from build123d import *

# Parameters (mm, degrees)
SKETCH1_W             = 203.2
SKETCH1_H             = 127
BOSS_EXTRUDE1_DEPTH   = 6.35
SKETCH2_W             = 196.85
SKETCH2_H             = 120.65
CUT_EXTRUDE1_DEPTH    = 7.35
SKETCH4_W             = 234.95
SKETCH4_H             = 158.75
SKETCH4_W_2           = 203.2
SKETCH4_H_2           = 127
BOSS_EXTRUDE2_DEPTH   = 6.35
SKETCH7_W             = 215.6206
SKETCH7_H             = 139.4206
SKETCH7_W_2           = 206.375
SKETCH7_H_2           = 130.175
CUT_EXTRUDE2_DEPTH    = 2.6416
F_8_32_TAPPED_HOLE1_D = 3.4544
FILLET3_R             = 4.6228
FILLET4_R             = 9.2456
FILLET5_R             = 3.175
F_6_CLEARANCE_HOLE1_D = 3.7973
SKETCH18_W            = 203.2
SKETCH18_H            = 127
CUT_EXTRUDE3_DEPTH    = 3.175
FILLET6_R             = 3.175


with BuildPart() as part:
    # Sketch1 → Boss-Extrude1 (new body)
    with BuildSketch(Plane(origin=(0, 0, 0), x_dir=(1, 0, 0), z_dir=(0, 1, 0))):
        Rectangle(SKETCH1_W, SKETCH1_H)
    extrude(amount=BOSS_EXTRUDE1_DEPTH)

    # Sketch2 → Cut-Extrude1 (cut, through all)
    with BuildSketch(Plane(origin=(0, 6.35, 0), x_dir=(1, 0, 0), z_dir=(0, 1, 0))):
        Rectangle(SKETCH2_W, SKETCH2_H)
    extrude(amount=-CUT_EXTRUDE1_DEPTH, mode=Mode.SUBTRACT)

    # Sketch4 → Boss-Extrude2 (add)
    with BuildSketch(Plane(origin=(0, 6.35, 0), x_dir=(1, 0, 0), z_dir=(0, 1, 0))):
        Rectangle(SKETCH4_W, SKETCH4_H)
        Rectangle(SKETCH4_W_2, SKETCH4_H_2, mode=Mode.SUBTRACT)
    extrude(amount=-BOSS_EXTRUDE2_DEPTH)

    # Sketch7 → Cut-Extrude2 (cut)
    with BuildSketch(Plane(origin=(0, 6.35, 0), x_dir=(1, 0, 0), z_dir=(0, 1, 0))):
        Rectangle(SKETCH7_W, SKETCH7_H)
        Rectangle(SKETCH7_W_2, SKETCH7_H_2, mode=Mode.SUBTRACT)
    extrude(amount=-CUT_EXTRUDE2_DEPTH, mode=Mode.SUBTRACT)

    # #8-32 Tapped Hole1 (through all)
    with Locations(Plane(origin=(0, 6.35, 0), x_dir=(1, 0, 0), z_dir=(0, 1, 0))):
        with Locations((56.321325, 74.54265), (112.64265, 74.54265), (112.64265, 24.84755), (0, 74.54265), (112.64265, -24.84755), (112.64265, -74.54265), (56.321325, -74.54265), (0, -74.54265), (-56.321325, -74.54265), (-112.64265, -74.54265), (-112.64265, -24.84755), (-112.64265, 24.84755), (-112.64265, 74.54265), (-56.321325, 74.54265)):
            Hole(F_8_32_TAPPED_HOLE1_D / 2)

    # Fillet3
    fillet3_edges = [part.edges().sort_by_distance(p)[0] for p in [
        (-103.1875, 5.0292, -65.0875),
        (103.1875, 5.0292, -65.0875),
        (103.1875, 5.0292, 65.0875),
        (-103.1875, 5.0292, 65.0875),
    ]]
    fillet(fillet3_edges, radius=FILLET3_R)

    # Fillet4
    fillet4_edges = [part.edges().sort_by_distance(p)[0] for p in [
        (-107.8103, 5.0292, -69.7103),
        (107.8103, 5.0292, -69.7103),
        (107.8103, 5.0292, 69.7103),
        (-107.8103, 5.0292, 69.7103),
    ]]
    fillet(fillet4_edges, radius=FILLET4_R)

    # Fillet5
    fillet5_edges = [part.edges().sort_by_distance(p)[0] for p in [
        (-98.425, 3.175, -60.325),
        (98.425, 3.175, -60.325),
        (98.425, 3.175, 60.325),
        (-98.425, 3.175, 60.325),
    ]]
    fillet(fillet5_edges, radius=FILLET5_R)

    # #6 Clearance Hole1 (through all)
    with Locations(Plane(origin=(0, 0, 0), x_dir=(-1, 0, 0), z_dir=(0, -1, 0))):
        with Locations((-98.425, 74.54265), (-98.425, -74.54265), (98.425, -74.54265), (98.425, 74.54265)):
            Hole(F_6_CLEARANCE_HOLE1_D / 2)

    # Sketch18 → Cut-Extrude3 (cut)
    with BuildSketch(Plane.XZ):
        Rectangle(SKETCH18_W, SKETCH18_H)
    extrude(amount=-CUT_EXTRUDE3_DEPTH, mode=Mode.SUBTRACT)

    # Fillet6
    fillet6_edges = [part.edges().sort_by_distance(p)[0] for p in [
        (-101.6, 1.5875, -63.5),
        (-101.6, 1.5875, 63.5),
        (101.6, 1.5875, 63.5),
        (101.6, 1.5875, -63.5),
    ]]
    fillet(fillet6_edges, radius=FILLET6_R)


solid = part.part
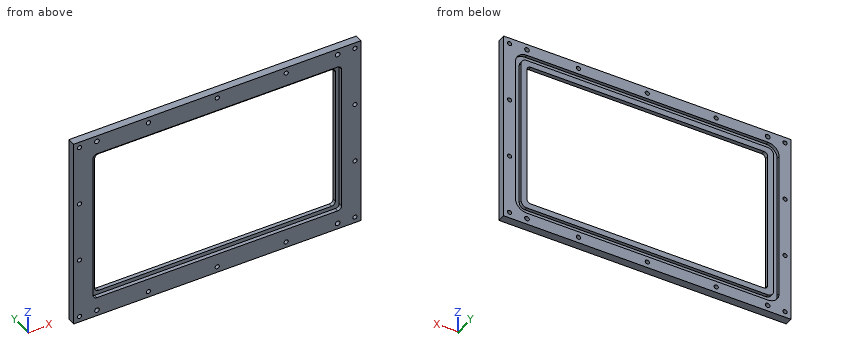
Here's how the part is built. I have some questions about the finished solid (model axes, mm). Give positions to 0.01 mm unless a question says otherwise; leave off trailing zeros. One line per item, written item: value.
Q1. I'm going to push flat-ended pins straight in: pin 1 Ø3 at (x, z) = (89.5, -57) entering from -Y; pin 2 Ø4.5 at (x, z) = (98.42, 74.54) entering from +Y. Where does each tip first touch, or does it pass through?
Answers follow:
pin 1: through
pin 2: y = 6.35
Q2. If I drill on line 1 along Z through (x, y) = (89.5, 4.25) (1 decimal); line 2 along Z through (x, y) = (0, 3.5) (3 decimals); line 3 along X through (y, z) = (4, 11) (1 decimal), over which ranges is the centre line in solid material (lowest first)?
Answers follow:
line 1: -79.4 to -69.7, -65.1 to -60.3, 60.3 to 65.1, 69.7 to 79.4
line 2: -79.375 to -76.27, -72.815 to -60.325, 60.325 to 72.815, 76.27 to 79.375
line 3: -117.5 to -107.8, -103.2 to -98.4, 98.4 to 103.2, 107.8 to 117.5
Q3. Suppose I cut it at C-C on y = 2. State how many separate pieces and enclosed holes the cut face has, then the cut area to 3 significant figures.
Answers follow:
separate pieces: 1
enclosed holes: 19
area: 11,300 mm^2
